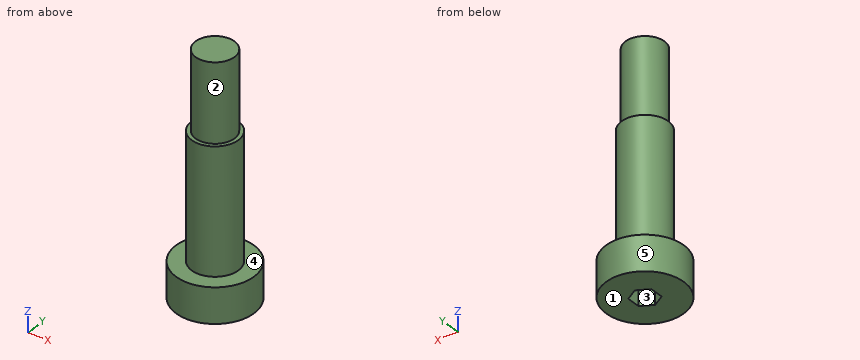
```python
from build123d import *

# Parameters (mm, degrees)
SKETCH_1_R          = 5
EXTRUDE_1_DEPTH     = 4.5
CUT_EXTRUDE_1_DEPTH = 2
SKETCH_3_R          = 3
EXTRUDE_2_DEPTH     = 16
SKETCH_4_R          = 2.5
EXTRUDE_3_DEPTH     = 10


with BuildPart() as part:
    # 草图1 → 凸台-拉伸1 (new body)
    with BuildSketch(Plane.XY):
        Circle(SKETCH_1_R)
    extrude(amount=EXTRUDE_1_DEPTH)

    # 草图2 → 切除-拉伸1 (cut)
    with BuildSketch(Plane(origin=(0, 0, 0), x_dir=(-1, 0, 0), z_dir=(0, 0, -1))):
        Polygon((1.5, -0.866025404), (1.5, 0.866025404), (0, 1.732050808), (-1.5, 0.866025404), (-1.5, -0.866025404), (0, -1.732050808), align=None)
    extrude(amount=-CUT_EXTRUDE_1_DEPTH, mode=Mode.SUBTRACT)

    # 草图3 → 凸台-拉伸2 (add)
    with BuildSketch(Plane.XY.offset(4.5)):
        Circle(SKETCH_3_R)
    extrude(amount=EXTRUDE_2_DEPTH)

    # 草图4 → 凸台-拉伸3 (add)
    with BuildSketch(Plane.XY.offset(20.5)):
        Circle(SKETCH_4_R)
    extrude(amount=EXTRUDE_3_DEPTH)


solid = part.part
```
Geometry: final body of the model. Coordinates: model frame, mm. Face numbers are marked on the shaded views. A direction names the side the tool comes from. Coordinates: 2 decimals unless noted, no trailing zeros. Order: outer loops, then holes, each group sorted by start corner. A loop starts at its lowest first (then second) coordinate and runs counter-clockwise, first axis right, second up.
Item 1: Section query B-B (z = 26.5). Output: boundary loops of the cut face in (x, y).
Answer:
outline: circle Ø5 at (0, 0)
Item 2: Section query A-A (y = 0). Output: boundary loops of the cut face in (x, z), then the cut area to 3 significant figures.
Answer:
outline: (-5, 0) - (-1.5, 0) - (-1.5, 2) - (1.5, 2) - (1.5, 0) - (5, 0) - (5, 4.5) - (3, 4.5) - (3, 20.5) - (2.5, 20.5) - (2.5, 30.5) - (-2.5, 30.5) - (-2.5, 20.5) - (-3, 20.5) - (-3, 4.5) - (-5, 4.5) - close
area: 185 mm2
Item 3: Material intervals for line 1 along X through (y, z) = (-4, 4); line 2 along Z through (x, y) = (2.5, -1.25); line 3 along Z through (x, y) = (-2.25, 3.75), sorted ascending.
Answer:
line 1: x = -3 to 3
line 2: z = 0 to 20.5
line 3: z = 0 to 4.5
Item 4: Draft query along Y for the marked faces 3, 4 and 5. Return one class per face: released by +Y, released by -Y, zero draft, split by the parting line, or undercut.
Answer:
face 3: undercut
face 4: zero draft
face 5: split by the parting line
Item 5: Section query D-D (x = 4). Output: boundary loops of the cut face in (y, z), then the cut area to 3 significant figures.
Answer:
outline: (-3, 0) - (3, 0) - (3, 4.5) - (-3, 4.5) - close
area: 27.0 mm2
Item 6: Contact query for flat-ended pins moving along their axis: P1, Ø0.5, axis at y = -0.5, z = 1, coming from the +X side; P2, Ø5, axis at x = 0.5, z = 24, coming from the -Y side; P3, Ø1.4, axis at y = 0.5, z = 0.5, coming from the -X side; P4, Ø5, axis at x = -3.5, z = 13.5, coming from the +Y side. Output: stop coordinate, or through.
Answer:
P1: stops at x = 4.99
P2: stops at y = -2.5
P3: stops at x = -5
P4: stops at y = 2.83
Item 7: Section query C-C (x = 1). Output: boundary loops of the cut face in (y, z).
Answer:
outline: (-4.9, 0) - (-1.15, 0) - (-1.15, 2) - (1.15, 2) - (1.15, 0) - (4.9, 0) - (4.9, 4.5) - (2.83, 4.5) - (2.83, 20.5) - (2.29, 20.5) - (2.29, 30.5) - (-2.29, 30.5) - (-2.29, 20.5) - (-2.83, 20.5) - (-2.83, 4.5) - (-4.9, 4.5) - close
Item 8: Access query for the marked faces 1 and 2. Directions: +Z, -Z, +X, -X, +Y, -Y. A direction counts if a zero-diameter tool reaches every point of the face in a straight line with its end or side. Return the directions, or none.
Answer:
face 1: -Z, +X, -X, +Y, -Y
face 2: +Z
